Drawing for the job (mm, zero at the part's lowest x, y, z). A direction names the side the tool comes from. Round coordinates to 2 decimals unless told otherwise and drop trailing zeros. Write each loop counter-clockwise with the first axis right and the second up, starting at its lowest first coordinate (ties: lowest second). Pieces come first, ordered by that corner, then holes.
Item 1: Band-saw the part on C-C, the plane x = 41.5. Write the cut outline in (y, z), then the cut area to 3 significant figures.
Item 2: Drop flat-ended pins along their axis: pin 1 Ø0.8 at (y, z) = (37.5, 14.5) entering from +X (3 decimals); pin 2 Ø7.5 at (x, z) = (21, 14) entering from +Y; pin 3 Ø6.5 at (x, z) = (48, 13) entering from +Y. Give the stop position or say it passes through.
Item 3: Band-saw the part on B-B, the plane z = 15. Write the cut outline in (x, y) (1 decimal).
Item 4: Wall check: probe 1 along X at (y, z) = (57, 22) (1 decimal); probe 2 along Y at (x, z) = (33, 7.25); probe 3 along Y at (x, z) = (49, 15.5). Give the ranges that are in metal, low to high.
Item 5: Band-saw the part on D-D, the plane x = 29.5. Write the cut outline in (y, z).
Item 6: 3-axis set-ups, long thin cutter, end or side, ignore diameter. For the marked faces 5, 6 and 7: which of +Z, -Z, +X, -X, +Y, -Y reach the whole face in a straight line?
Item 7: Mould opens along X. For the marked faces 1, 2, 3 and 4 say: +X half, -X half, draft (parallel to the pull), parting line (faces both ways), or undercut.
Item 8: Band-saw the part on A-A, the plane y = 51. Count the separate pieces of the cut face and the enclosed holes in it, then the cut area to 3 significant figures.
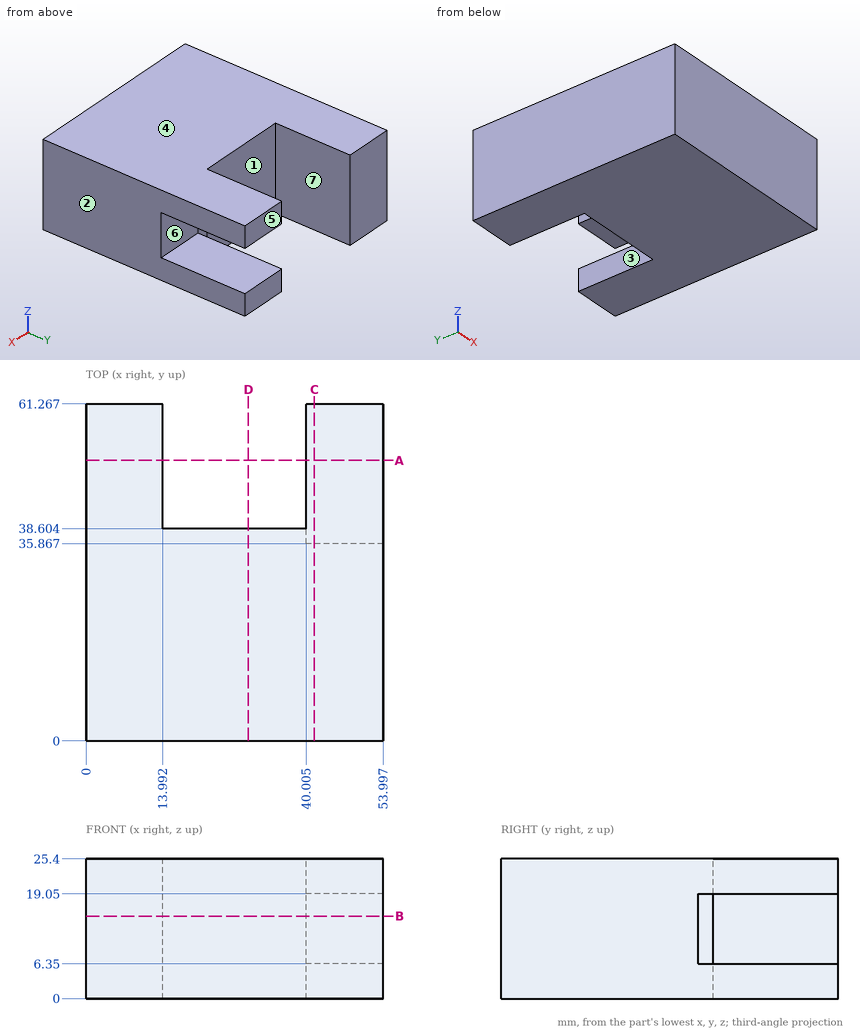
Results:
1. outline: (0, 0) - (61.27, 0) - (61.27, 6.35) - (35.87, 6.35) - (35.87, 19.05) - (61.27, 19.05) - (61.27, 25.4) - (0, 25.4) - close
1. area: 1,230 mm2
2. pin 1: stops at x = 40.005
2. pin 2: stops at y = 38.6
2. pin 3: stops at y = 35.87
3. outline: (0, 0) - (54, 0) - (54, 35.9) - (40, 35.9) - (40, 38.6) - (14, 38.6) - (14, 61.3) - (0, 61.3) - close
4. probe 1: x = 0 to 14, 40 to 54
4. probe 2: y = 0 to 38.6
4. probe 3: y = 0 to 35.87
5. outline: (0, 0) - (38.6, 0) - (38.6, 25.4) - (0, 25.4) - close
6. face 5: +Z, -Z, +X, -X, +Y
6. face 6: +X, +Y
6. face 7: +Z, -Z, +Y
7. face 1: undercut
7. face 2: +X half
7. face 3: undercut
7. face 4: draft
8. separate pieces: 3
8. enclosed holes: 0
8. area: 533 mm2
